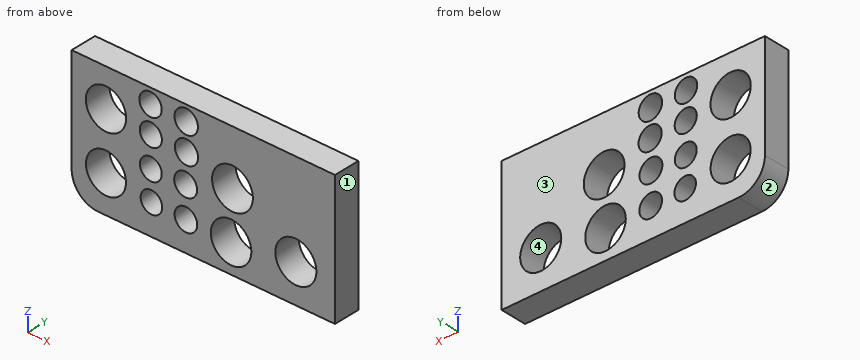
from build123d import *

# Parameters (mm, degrees)
SKETCH1_W              = 100
SKETCH1_H              = 50
BOSS_EXTRUDE1_DEPTH    = 10
FILLET1_R              = 10
F_1_0MM_DOWEL_HOLE1_D  = 15.2
F_1_0MM_DOWEL_HOLE2_D  = 15.3
F_1_0MM_DOWEL_HOLE3_D  = 8.2
F_1_0MM_DOWEL_HOLE4_D  = 8.3
F_1_0MM_DOWEL_HOLE5_D  = 8.4
F_1_0MM_DOWEL_HOLE6_D  = 8.5
F_1_0MM_DOWEL_HOLE7_D  = 8.6
F_1_0MM_DOWEL_HOLE8_D  = 8.7
F_1_0MM_DOWEL_HOLE9_D  = 8.8
F_1_0MM_DOWEL_HOLE10_D = 8.9
F_1_0MM_DOWEL_HOLE11_D = 15.4
F_1_0MM_DOWEL_HOLE12_D = 15.5
F_1_0MM_DOWEL_HOLE13_D = 15.6


with BuildPart() as part:
    # Sketch1 → Boss-Extrude1 (new body)
    with BuildSketch(Plane(origin=(0, 0, 0), x_dir=(1, 0, 0), z_dir=(0, 1, 0))):
        Rectangle(SKETCH1_W, SKETCH1_H)
    extrude(amount=BOSS_EXTRUDE1_DEPTH)

    # Fillet1
    fillet1_edges = [part.edges().sort_by_distance(p)[0] for p in [
        (-50, 5, -25),
    ]]
    fillet(fillet1_edges, radius=FILLET1_R)

    # Ø1.0mm Dowel Hole1 (through all)
    with Locations(Plane(origin=(0, 10, 0), x_dir=(1, 0, 0), z_dir=(0, 1, 0))):
        with Locations((-36.962140768, 10.811692473)):
            Hole(F_1_0MM_DOWEL_HOLE1_D / 2)

    # Ø1.0mm Dowel Hole2 (through all)
    with Locations(Plane(origin=(0, 10, 0), x_dir=(1, 0, 0), z_dir=(0, 1, 0))):
        with Locations((-36.962140768, -10.705173335)):
            Hole(F_1_0MM_DOWEL_HOLE2_D / 2)

    # Ø1.0mm Dowel Hole3 (through all)
    with Locations(Plane(origin=(0, 10, 0), x_dir=(1, 0, 0), z_dir=(0, 1, 0))):
        with Locations((-19.706040467, 13.368151776)):
            Hole(F_1_0MM_DOWEL_HOLE3_D / 2)

    # Ø1.0mm Dowel Hole4 (through all)
    with Locations(Plane(origin=(0, 10, 0), x_dir=(1, 0, 0), z_dir=(0, 1, 0))):
        with Locations((-19.919078743, 2.29016146)):
            Hole(F_1_0MM_DOWEL_HOLE4_D / 2)

    # Ø1.0mm Dowel Hole5 (through all)
    with Locations(Plane(origin=(0, 10, 0), x_dir=(1, 0, 0), z_dir=(0, 1, 0))):
        with Locations((-19.919078743, -9.213905408)):
            Hole(F_1_0MM_DOWEL_HOLE5_D / 2)

    # Ø1.0mm Dowel Hole6 (through all)
    with Locations(Plane(origin=(0, 10, 0), x_dir=(1, 0, 0), z_dir=(0, 1, 0))):
        with Locations((-20.02559788, -19.333223485)):
            Hole(F_1_0MM_DOWEL_HOLE6_D / 2)

    # Ø1.0mm Dowel Hole7 (through all)
    with Locations(Plane(origin=(0, 10, 0), x_dir=(1, 0, 0), z_dir=(0, 1, 0))):
        with Locations((-6.604186535, 13.687709189)):
            Hole(F_1_0MM_DOWEL_HOLE7_D / 2)

    # Ø1.0mm Dowel Hole8 (through all)
    with Locations(Plane(origin=(0, 10, 0), x_dir=(1, 0, 0), z_dir=(0, 1, 0))):
        with Locations((-6.710705673, 1.970604047)):
            Hole(F_1_0MM_DOWEL_HOLE8_D / 2)

    # Ø1.0mm Dowel Hole9 (through all)
    with Locations(Plane(origin=(0, 10, 0), x_dir=(1, 0, 0), z_dir=(0, 1, 0))):
        with Locations((-6.39114826, -9.000867132)):
            Hole(F_1_0MM_DOWEL_HOLE9_D / 2)

    # Ø1.0mm Dowel Hole10 (through all)
    with Locations(Plane(origin=(-6.497667397, 10, 19.226704348), x_dir=(0, 0, 1), z_dir=(0, 1, 0))):
        with Locations((0, 0)):
            Hole(F_1_0MM_DOWEL_HOLE10_D / 2)

    # Ø1.0mm Dowel Hole11 (through all)
    with Locations(Plane(origin=(0, 10, 0), x_dir=(1, 0, 0), z_dir=(0, 1, 0))):
        with Locations((10.545394628, 14.11378574)):
            Hole(F_1_0MM_DOWEL_HOLE11_D / 2)

    # Ø1.0mm Dowel Hole12 (through all)
    with Locations(Plane(origin=(0, 10, 0), x_dir=(1, 0, 0), z_dir=(0, 1, 0))):
        with Locations((11.077990317, -4.1009868)):
            Hole(F_1_0MM_DOWEL_HOLE12_D / 2)

    # Ø1.0mm Dowel Hole13 (through all)
    with Locations(Plane(origin=(0, 10, 0), x_dir=(1, 0, 0), z_dir=(0, 1, 0))):
        with Locations((35.151315428, 10.385615922)):
            Hole(F_1_0MM_DOWEL_HOLE13_D / 2)


solid = part.part
Build history of the part. All positions in model axes, mm. Face numbers are marked on the shaded views. Coordinates: 2 decimals unless noted, no trailing zeros. Write each loop counter-clockwise with the first axis right and the second up, starting at its lowest first coordinate (ties: lowest second). Pieces come first, ordered by that corner, then holes.
(1) Drill centre lines: line 1 (X direction, y = 2.25, z = 19); line 2 (X direction, y = 1.75, z = 10); line 3 (Z direction, x = 5, y = 4.75). Where is each one in solid material? Low to high.
(2) Cut at A-A on x = -41.5. List the corners of the cut face in (y, z).
(3) Mould opens along X. For the marked faces 1, 2, 3 and 4 say: pulls with the +X half, pulls with the -X half, needs draft (parallel to the pull), parting line crosses it, or undercut.
(4) Cut at B-B on z = 21. List the corners of the cut face in (x, y).
(5) Cut at D-D on z = -8. List the corners of the cut face in (x, y), and give its area (3 significant figures).
(6) Pin check, flat tip, straight feed: pin 1 Ø9.5 at (x, z) = (35.15, -10.39) entering from -Y. Stop position of the tip, or through.
(7) Cut at C-C on x = 31. List the corners of the cut face in (y, z), and give its area (3 significant figures).
Working result:
1. line 1: x = -50 to -24.26, -15.79 to -10.94, -2.05 to 50
1. line 2: x = -50 to -44.58, -29.34 to -24.04, -15.79 to -10.68, -2.11 to 6.05, 16.1 to 50
1. line 3: z = -25 to -19.46, -8.77 to -0.71, 8.91 to 25
2. outline: (0, -24.89) - (10, -24.89) - (10, -16.91) - (0, -16.91) - close; (0, -4.72) - (10, -4.72) - (10, 4.55) - (0, 4.55) - close; (0, 16.86) - (10, 16.86) - (10, 25) - (0, 25) - close
3. face 1: pulls with the +X half
3. face 2: pulls with the -X half
3. face 3: needs draft
3. face 4: undercut
4. outline: (-50, 0) - (-23.94, 0) - (-23.94, 10) - (-50, 10) - close; (-16.12, 0) - (-10.58, 0) - (-10.58, 10) - (-16.12, 10) - close; (-2.42, 0) - (50, 0) - (50, 10) - (-2.42, 10) - close
5. outline: (-50, 0) - (-44.02, 0) - (-44.02, 10) - (-50, 10) - close; (-29.9, 0) - (5.86, 0) - (5.86, 10) - (-29.9, 10) - close; (15.23, 0) - (27.73, 0) - (27.73, 10) - (15.23, 10) - close; (42.58, 0) - (50, 0) - (50, 10) - (42.58, 10) - close
5. area: 617 mm2
6. pin 1: passes through
7. outline: (0, -25) - (10, -25) - (10, -16.99) - (0, -16.99) - close; (0, -3.78) - (10, -3.78) - (10, 25) - (0, 25) - close
7. area: 368 mm2
